from build123d import *

# Parameters (mm, degrees)
SKETCH1_W           = 33.814565048
SKETCH1_H           = 35.83261461
BOSS_EXTRUDE1_DEPTH = 8
SKETCH2_R           = 1.75
CUT_EXTRUDE1_DEPTH  = 8
SKETCH3_R           = 2.25
CUT_EXTRUDE2_DEPTH  = 10
CHAMFER1_SIZE       = 4
CUT_EXTRUDE3_DEPTH  = 3


with BuildPart() as part:
    # Sketch1 → Boss-Extrude1 (new body)
    with BuildSketch(Plane.XY):
        Rectangle(SKETCH1_W, SKETCH1_H)
    extrude(amount=BOSS_EXTRUDE1_DEPTH)

    # Sketch2 → Cut-Extrude1 (cut)
    with BuildSketch(Plane.XY.offset(8)):
        with Locations((-12, 0)):
            Circle(SKETCH2_R)
        with Locations((12, 0)):
            Circle(SKETCH2_R)
    extrude(amount=-CUT_EXTRUDE1_DEPTH, mode=Mode.SUBTRACT)

    # Sketch3 → Cut-Extrude2 (cut)
    with BuildSketch(Plane(origin=(0, 0, 0), x_dir=(-1, 0, 0), z_dir=(0, 0, -1))):
        with Locations((11.5, -11.5)):
            Circle(SKETCH3_R)
        with Locations((-11.5, -11.5)):
            Circle(SKETCH3_R)
        with Locations((-11.5, 11.5)):
            Circle(SKETCH3_R)
        with Locations((11.5, 11.5)):
            Circle(SKETCH3_R)
    extrude(amount=-CUT_EXTRUDE2_DEPTH, mode=Mode.SUBTRACT)

    # Chamfer1
    chamfer1_edges = [part.edges().sort_by_distance(p)[0] for p in [
        (-16.907282524, 17.916307305, 4),
        (16.907282524, 17.916307305, 4),
        (16.907282524, -17.916307305, 4),
        (-16.907282524, -17.916307305, 4),
    ]]
    chamfer(chamfer1_edges, length=CHAMFER1_SIZE)

    # Sketch4 → Cut-Extrude3 (cut)
    with BuildSketch(Plane(origin=(0, 0, 0), x_dir=(-1, 0, 0), z_dir=(0, 0, -1))):
        Polygon((-12, -3.550704156), (-8.925, -1.775352078), (-8.925, 1.775352078), (-12, 3.550704156), (-15.075, 1.775352078), (-15.075, -1.775352078), align=None)
        Polygon((12, -3.550704156), (15.075, -1.775352078), (15.075, 1.775352078), (12, 3.550704156), (8.925, 1.775352078), (8.925, -1.775352078), align=None)
    extrude(amount=-CUT_EXTRUDE3_DEPTH, mode=Mode.SUBTRACT)


solid = part.part
Check sheet for the modelled part. Datum: model origin and axes. Units: mm. A direction names the side the tool comes from. Coordinates: 2 decimals unless noted, no trailing zeros. Loops run counter-clockwise (first coordinate to the right, second up) from the corner with the lowest first, then second, coordinate; pieces in that order, holes last. Notation, with made-up numbers: (87, -32) -> (107, -32) arc R29 cw to (107, 4) -> close; hole circle Ø9 at (-30.75, 58.25). An arc over 180 degrees is marked (long way). Write item = value, one per line. Start each with the question number.
1. Section check C-C on x = -11. Record the cut outline in (y, z), then the cut area to 3 significant figures.
2. Material ranges on line 1 (X direction, y = -12.5, z = 1.75); line 2 (X direction, y = 3, z = 2); line 3 (Y direction, x = -12, z = 6.8), recorded low to high.
3. Section check A-A on z = 6.5. Record the cut outline in (x, y).
4. Section check D-D on y = 0. Record the cut outline in (x, z) (3 decimals).
5. Section check B-B on y = -11.5. Record the cut outline in (x, z), then the cut area to 3 significant figures.
6. Depth check by flat-ended pin: P1, Ø6, axis at x = -13, y = 12, coming from the -Z side; P2, Ø3, axis at x = -12, y = 1, coming from the -Z side. Enter the tip coordinate at first touch or a pass-through.
7. Tool access check on faces 4 (the cylindrical face through (13.16, 13.02, 3.94)), 5 (the flat face through (15.075, 0, 1)). Record the directions out of +Z, -Z, +X, -X, +Y, -Y that give a thin tool (end or side, any length) a straight path to the whole face; none if there is none.
8. Draft check along X on faces 1 (the flat face through (-14.879, 15.944, 3.944)), 2 (the flat face through (10.44, 2.65, 1.48)), 3 (the flat face through (0, 17.916, 4)). Enter one of: released by +X, released by -X, zero draft, split by the parting line, or undercut.
Responses:
q1.outline = (-17.92, 0) -> (-13.69, 0) -> (-13.69, 8) -> (-17.92, 8) -> close; (-9.31, 0) -> (-2.97, 0) -> (-2.97, 3) -> (-1.44, 3) -> (-1.44, 8) -> (-9.31, 8) -> close; (1.44, 3) -> (2.97, 3) -> (2.97, 0) -> (9.31, 0) -> (9.31, 8) -> (1.44, 8) -> close; (13.69, 0) -> (17.92, 0) -> (17.92, 8) -> (13.69, 8) -> close
q1.area = 184 mm2
q2.line_1 = -16.91 to -13.52, -9.48 to 9.48, 13.52 to 16.91
q2.line_2 = -16.91 to -12.95, -11.05 to 11.05, 12.95 to 16.91
q2.line_3 = -17.92 to -13.69, -9.31 to -1.75, 1.75 to 9.31, 13.69 to 17.92
q3.outline = (-16.91, -13.92) -> (-12.91, -17.92) -> (12.91, -17.92) -> (16.91, -13.92) -> (16.91, 13.92) -> (12.91, 17.92) -> (-12.91, 17.92) -> (-16.91, 13.92) -> close; hole circle Ø4.5 at (-11.5, -11.5); hole circle Ø3.5 at (-12, 0); hole circle Ø4.5 at (-11.5, 11.5); hole circle Ø4.5 at (11.5, -11.5); hole circle Ø4.5 at (11.5, 11.5); hole circle Ø3.5 at (12, 0)
q4.outline = (-16.907, 0) -> (-15.075, 0) -> (-15.075, 3) -> (-13.75, 3) -> (-13.75, 8) -> (-16.907, 8) -> close; (-10.25, 3) -> (-8.925, 3) -> (-8.925, 0) -> (8.925, 0) -> (8.925, 3) -> (10.25, 3) -> (10.25, 8) -> (-10.25, 8) -> close; (13.75, 3) -> (15.075, 3) -> (15.075, 0) -> (16.907, 0) -> (16.907, 8) -> (13.75, 8) -> close
q5.outline = (-16.91, 0) -> (-13.75, 0) -> (-13.75, 8) -> (-16.91, 8) -> close; (-9.25, 0) -> (9.25, 0) -> (9.25, 8) -> (-9.25, 8) -> close; (13.75, 0) -> (16.91, 0) -> (16.91, 8) -> (13.75, 8) -> close
q5.area = 199 mm2
q6.P1 = 0
q6.P2 = 3
q7.face_4 = +Z, -Z
q7.face_5 = -Z
q8.face_1 = released by -X
q8.face_2 = undercut
q8.face_3 = zero draft
